```python
from build123d import *

# Parameters (mm, degrees)
SKETCH1_W           = 30
SKETCH1_H           = 37.25
BOSS_EXTRUDE1_DEPTH = 6
SKETCH2_R           = 2
CUT_EXTRUDE1_DEPTH  = 6
SKETCH3_W           = 10
SKETCH3_H           = 37.25
BOSS_EXTRUDE2_DEPTH = 4
SKETCH4_W           = 8
SKETCH4_H           = 37.25
CUT_EXTRUDE2_DEPTH  = 6
FILLET2_R           = 4
FILLET3_R           = 4
CUT_EXTRUDE3_DEPTH  = 50


with BuildPart() as part:
    # Sketch1 → Boss-Extrude1 (new body)
    with BuildSketch(Plane(origin=(0, 0, 0), x_dir=(1, 0, 0), z_dir=(0, 1, 0))):
        with Locations((2.786458333, -10.239583333)):
            Rectangle(SKETCH1_W, SKETCH1_H)
    extrude(amount=BOSS_EXTRUDE1_DEPTH)

    # Sketch2 → Cut-Extrude1 (cut)
    with BuildSketch(Plane(origin=(0, 6, 0), x_dir=(1, 0, 0), z_dir=(0, 1, 0))):
        with Locations(Location((-8.213541667, -24.864583333, 0), (0, 0, 270))):
            Circle(SKETCH2_R)
        with Locations(Location((11.786458333, 4.385416667, 0), (0, 0, 270))):
            Circle(SKETCH2_R)
        with Locations(Location((11.786458333, -24.864583333, 0), (0, 0, 270))):
            Circle(SKETCH2_R)
        with Locations(Location((-8.213541667, 4.385416667, 0), (0, 0, 270))):
            Circle(SKETCH2_R)
    extrude(amount=-CUT_EXTRUDE1_DEPTH, mode=Mode.SUBTRACT)

    # Sketch3 → Boss-Extrude2 (add)
    with BuildSketch(Plane(origin=(0, 6, 0), x_dir=(1, 0, 0), z_dir=(0, 1, 0))):
        with Locations((2.786458333, -10.239583333)):
            Rectangle(SKETCH3_W, SKETCH3_H)
    extrude(amount=BOSS_EXTRUDE2_DEPTH)

    # Sketch4 → Cut-Extrude2 (cut)
    with BuildSketch(Plane.XZ):
        with Locations((2.786458333, 10.239583333)):
            Rectangle(SKETCH4_W, SKETCH4_H)
    extrude(amount=-CUT_EXTRUDE2_DEPTH, mode=Mode.SUBTRACT)

    # Fillet2
    fillet2_edges = [part.edges().sort_by_distance(p)[0] for p in [
        (6.786458333, 6, 10.239583333),
        (-1.213541667, 6, 10.239583333),
    ]]
    fillet(fillet2_edges, radius=FILLET2_R - 0.0001)  # a hair under: the kernel refuses the full size

    # Fillet3
    fillet3_edges = [part.edges().sort_by_distance(p)[0] for p in [
        (7.786458333, 10, 10.239583333),
        (-2.213541667, 10, 10.239583333),
    ]]
    fillet(fillet3_edges, radius=FILLET3_R - 0.0001)  # a hair under: the kernel refuses the full size

    # Sketch5 → Cut-Extrude3 (cut)
    with BuildSketch(Plane(origin=(0, 0, -8.385416667), x_dir=(-1, 0, 0), z_dir=(0, 0, -1))):
        Polygon((-17.786458333, 0), (-17.085914813, 6), (-17.786458333, 6), align=None)
    extrude(amount=-CUT_EXTRUDE3_DEPTH, mode=Mode.SUBTRACT)


solid = part.part
```
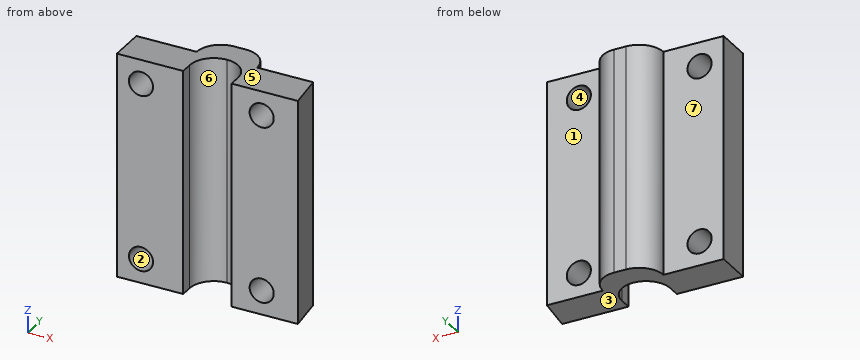
Could you check a few things on this model? Use its own coordinates, in mm. Face numbers are marked on the shaded views. A direction names the side the tool comes from. Coordinates: 2 decimals unless noted, no trailing zeros. Write each loop counter-clockwise with the first axis right and the second up, starting at its lowest first coordinate (ties: lowest second). Pieces come first, ordered by that corner, then holes. Notation, with made-up numbers: M -23.5,-30 L 3.5,-30 A20 ccw 3.5,-25 Z; hole C 80.25,8 d4. An arc over 180 degrees is marked long. Answer as CSV lines item,"result". Start each with the question number.
1) I want a section at C-C, the plane z = 24. Give the number of separate pieces and of enclosed holes in the cut face, and give its area (3 significant figures).
2) Please list where these lines run through material, in increasing order: line 1 (Z direction, x = -8.25, y = 2); line 2 (X direction, y = 4.75, z = -3.5); line 3 (X direction, y = 3.5, z = -3). Write a range as from..to.
3) For P1, Ø1, axis at y = 8.5, z = 15.5, coming from the -X side; P2, Ø3, axis at x = -6, z = 12.5, coming from the +Y side; P3, Ø2, axis at x = 1.5, z = 19, coming from the -Y side, each with a flat end and sliding along its axis, tell me the tip position at first contact or that it passes through.
4) I want a section at A-A, the plane y = 2.75. Please give me the cut outline in (x, z).
5) We'd pull the mould along Z, two halves only. Please class the marked faces 1, 2, 3 and 4: +Z half, -Z half, draft (parallel to the pull), parting line (faces both ways), or undercut.
6) I want a section at B-B, the plane x = -7.25. Please give me the cut outline in (y, z), and give its area (3 significant figures).
7) For the marked faces 5, 6 and 7, which set-ups out of +Z, -Z, +X, -X, +Y, -Y let a thin tool reach every point of the face, with its end or its side?
Data:
1,separate pieces,"3"
1,enclosed holes,"0"
1,area,"127 mm^2"
2,line 1,"z = -8.39..-6.39, -2.39..22.86, 26.86..28.86"
2,line 2,"x = -12.21..-10.01, -6.42..-0.12, 5.69..9.99, 13.58..17.23"
2,line 3,"x = -12.21..-9.66, -6.77..-0.92, 6.49..10.34, 13.23..17.38"
3,P1,"stops at x = -1.68"
3,P2,"stops at y = 6"
3,P3,"stops at y = 5.28"
4,outline,"M -12.21,-8.39 L -1.14,-8.39 L -1.14,28.86 L -12.21,28.86 Z; M 6.72,-8.39 L 17.47,-8.39 L 17.47,28.86 L 6.72,28.86 Z; hole C -8.21,-4.39 d4; hole C -8.21,24.86 d4; hole C 11.79,-4.39 d4; hole C 11.79,24.86 d4"
5,face 1,"draft"
5,face 2,"undercut"
5,face 3,"-Z half"
5,face 4,"undercut"
6,outline,"M 0,-8.39 L 6,-8.39 L 6,-6.14 L 0,-6.14 Z; M 0,-2.63 L 6,-2.63 L 6,23.11 L 0,23.11 Z; M 0,26.62 L 6,26.62 L 6,28.86 L 0,28.86 Z"
6,area,"181 mm^2"
7,face 5,"+Z, +X, -X, +Y, -Y"
7,face 6,"+Z, -Z, -Y"
7,face 7,"+Z, -Z, -X, +Y"
